Input: dimensioned drawing with shaded views. Units: mm. Origin: part minimum x, y, z. A direction names the side the tool comes from. Coordinates: 2 decimals unless noted, no trailing zeros. Order: outer loops, then holes, each group sorted by start corner. A loop starts at its lowest first (then second) coordinate and runs counter-clockwise, first axis right, second up. Notation, with made-up numbers: (-11, 35.5) - (39, 35.5) arc R8 ccw to (39, 41.5) - close; hole circle Ø10 at (87, -31). An arc over 180 degrees is marked (long way). Answer as CSV lines item,"result". Start each with the question number.
Item 1: Section A-A (z = 3). Output: boundary loops of the cut face in (x, y).
Item 2: Material intervals for line 1 along Y through (x, z) = (15.25, 3.1); line 2 along X through (y, z) = (3, 2.2); line 3 along Z through (x, y) = (4, 1.15), sorted ascending.
Item 3: First-contact query: pin 1 (1.5 mm diameter, centred on x = 2, z = 4, fed in from +Y); pin 2 (0.9 mm diameter, centred on x = 2, z = 4, fed in from -Y). Flat tips, straight axial feed; report the tip coordinate or a pass-through.
Item 4: Section B-B (y = 3). Output: boundary loops of the cut face in (x, z).
Item 5: Section C-C (x = 15.25). Output: boundary loops of the cut face in (y, z).
Item 6: Access query for the marked faces 1 and 2. Directions: +Z, -Z, +X, -X, +Y, -Y. A direction counts if a zero-diameter tool reaches every point of the face in a straight line with its end or side. Return the directions, or none.
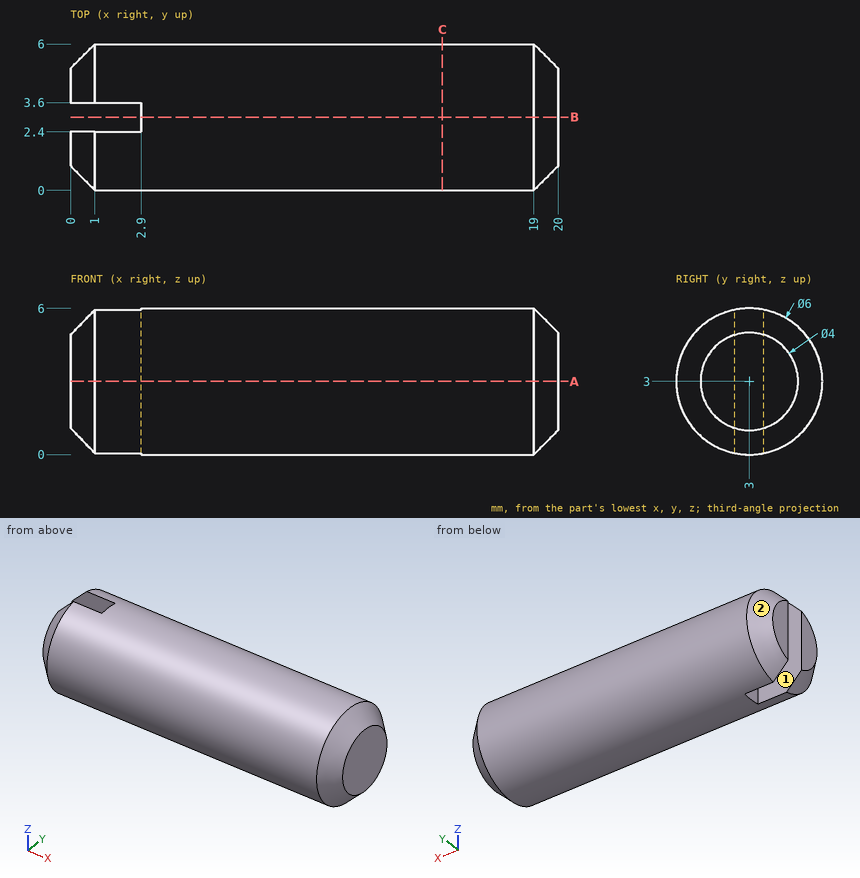
Determined:
1,outline,"(0, 1) - (1, 0) - (19, 0) - (20, 1) - (20, 5) - (19, 6) - (1, 6) - (0, 5) - (0, 3.6) - (2.9, 3.6) - (2.9, 2.4) - (0, 2.4) - close"
2,line 1,"y = 0 to 6"
2,line 2,"x = 2.9 to 20"
2,line 3,"z = 0.64 to 5.36"
3,pin 1,"stops at y = 5.99"
3,pin 2,"stops at y = 0.05"
4,outline,"(2.9, 0) - (19, 0) - (20, 1) - (20, 5) - (19, 6) - (2.9, 6) - close"
5,outline,"circle Ø6 at (3, 3)"
6,face 1,"+Z, -Z, -X"
6,face 2,"-X, +Y"
